Check sheet for the modelled part. Datum: model origin and axes. Units: mm. A direction names the side the tool comes from. Coordinates: 2 decimals unless noted, no trailing zeros. Loops run counter-clockwise (first coordinate to the right, second up) from the corner with the lowest first, then second, coordinate; pieces in that order, holes last. Notation, with made-up numbers: M 73,43.5 L 82,43.5 A31 cw 82,81.5 Z; hole C 29.5,34.25 d3. An arc over 180 degrees is marked long. Use CSV: the item, a comma, the result in double quotes. Start each with the question number.
(1) Set-up check for faces 5 (the flat face through (-16, -13, -6)), 6 (the cylindrical face through (-19.334, -1.014, -2.539)): record each of +Z, -Z, +X, -X, +Y, -Y from which the full face is reachable in a straight line by a thin tool's end or side.
(2) Section check A-A on z = 0. Record the cut outline in (x, y) (3 decimals).
(3) Section check D-D on z = 11. Record the cut outline in (x, y), and give its area (3 significant figures).
(4) Scan lines: line 1 (Y direction, x = 14, z = 9.5); line 2 (X direction, y = -4, z = 0) (3 decimals); line 3 (X direction, y = -1.5, z = -12.5). Record each from-to range of solid material in increasing order.
(5) Section check B-B on x = 0. Record the cut outline in (y, z) (3 decimals), and give its area (3 significant figures).
(6) Go/stop test with flat-tipped pins: pin 1 Ø1 at (x, y) = (-5, -7) entering from -Z; pin 2 Ø5 at (x, y) = (5, -6.5) entering from -Z; pin 3 Ø1 at (y, z) = (-5.5, 8) entering from +X. Record where each tip stops, or that it passes through.
(7) Draft check along Y on faces 1 (the flat face through (4, 0, 0)), 2 (the flat face through (4, -15, 0)), 3 (the cylindrical face through (-16.66, -7.58, -2.19)), 4 (the flat face through (-16, -2, 6)). Enter one of: pulls with the +Y half, pulls with the -Y half, needs draft (parallel to the pull), parting line crosses it, or undercut.
(8) Section check C-C on y = -9. Record the cut outline in (x, z) (3 decimals).
from build123d import *

# Parameters (mm, degrees)
SKETCH_2_R          = 3
CUT_EXTRUDE_1_DEPTH = 32.392674305


with BuildPart() as part:
    # 草图1 → 旋转1 (revolve)
    with BuildSketch(Plane.XY, mode=Mode.PRIVATE) as revolve_1_sk:
        Polygon((0, 0), (19.5, 0), (19.5, -2), (16.805, -2), (16.805, -13), (19.5, -13), (19.5, -15), (0, -15), align=None)
    revolve(revolve_1_sk.sketch.rotate(Axis((0, 23.575757576, 0), (0, -1, 0)), 90), axis=Axis((0, 23.575757576, 0), (0, -1, 0)))

    # 草图2 → 切除-拉伸1 (cut, through all)
    with BuildSketch(Plane(origin=(0, 0, 0), x_dir=(1, 0, 0), z_dir=(0, 1, 0))):
        with Locations(Location((0, 0, 0), (0, 0, 270))):
            Circle(SKETCH_2_R)
    extrude(amount=-CUT_EXTRUDE_1_DEPTH, mode=Mode.SUBTRACT)


solid = part.part
Outcome:
1,face 5,"none"
1,face 6,"+Y, -Y"
2,outline,"M -19.5,-15 L -3,-15 L -3,0 L -19.5,0 L -19.5,-2 L -16.805,-2 L -16.805,-13 L -19.5,-13 Z; M 3,-15 L 19.5,-15 L 19.5,-13 L 16.805,-13 L 16.805,-2 L 19.5,-2 L 19.5,0 L 3,0 Z"
3,outline,"M -16.1,-15 L 16.1,-15 L 16.1,-13 L 12.7,-13 L 12.7,-2 L 16.1,-2 L 16.1,0 L -16.1,0 L -16.1,-2 L -12.7,-2 L -12.7,-13 L -16.1,-13 Z"
3,area,"408 mm²"
4,line 1,"y = -15 to -13, -2 to 0"
4,line 2,"x = -16.805 to -3, 3 to 16.805"
4,line 3,"x = -14.97 to 14.97"
5,outline,"M -15,-19.5 L -13,-19.5 L -13,-16.805 L -2,-16.805 L -2,-19.5 L 0,-19.5 L 0,-3 L -15,-3 Z; M -15,3 L 0,3 L 0,19.5 L -2,19.5 L -2,16.805 L -13,16.805 L -13,19.5 L -15,19.5 Z"
5,area,"436 mm²"
6,pin 1,"stops at z = -16.19"
6,pin 2,"stops at z = -16.62"
6,pin 3,"stops at x = 15.04"
7,face 1,"pulls with the +Y half"
7,face 2,"pulls with the -Y half"
7,face 3,"undercut"
7,face 4,"undercut"
8,outline,"C 0,0 d33.61; hole C 0,0 d6"
